Geometry check sheet. Reference: drawing and pictorial views, mm from the part's lowest x, y, z. Round coordinates to 2 decimals unless told otherwise and drop trailing zeros. Order: outer loops, then holes, each group sorted by start corner. A loop starts at its lowest first (then second) coordinate and runs counter-clockwise, first axis right, second up.
(1) Go/stop test with flat-tipped pins: pin 1 (1.8 mm diameter, centred on x = 84, y = 2.5, fed in from -Z); pin 2 (1.8 mm diameter, centred on y = 4, z = 54.5, fed in from -X); pin 3 (1.5 mm diameter, centred on x = 45.5, y = 5, fed in from +Z). Record where each tip stops, or that it passes through.
(2) Sectioned sample at C-C (x = 31). Record the boundary of the cut face in (y, z), plus the area to 3 significant figures.
(3) Material ranges on line 1 along Z through (x, y) = (5, 4); line 2 along X through (y, z) = (2.8, 63.5); line 3 along Z through (x, y) = (51, 1.6), recorded low to high.
(4) Sectioned sample at A-A (y = 2.35). Record the boundary of the cut face in (x, z).
(5) Sectioned sample at B-B (z = 59). Record the boundary of the cut face in (x, y), plus the area to 3 significant figures.
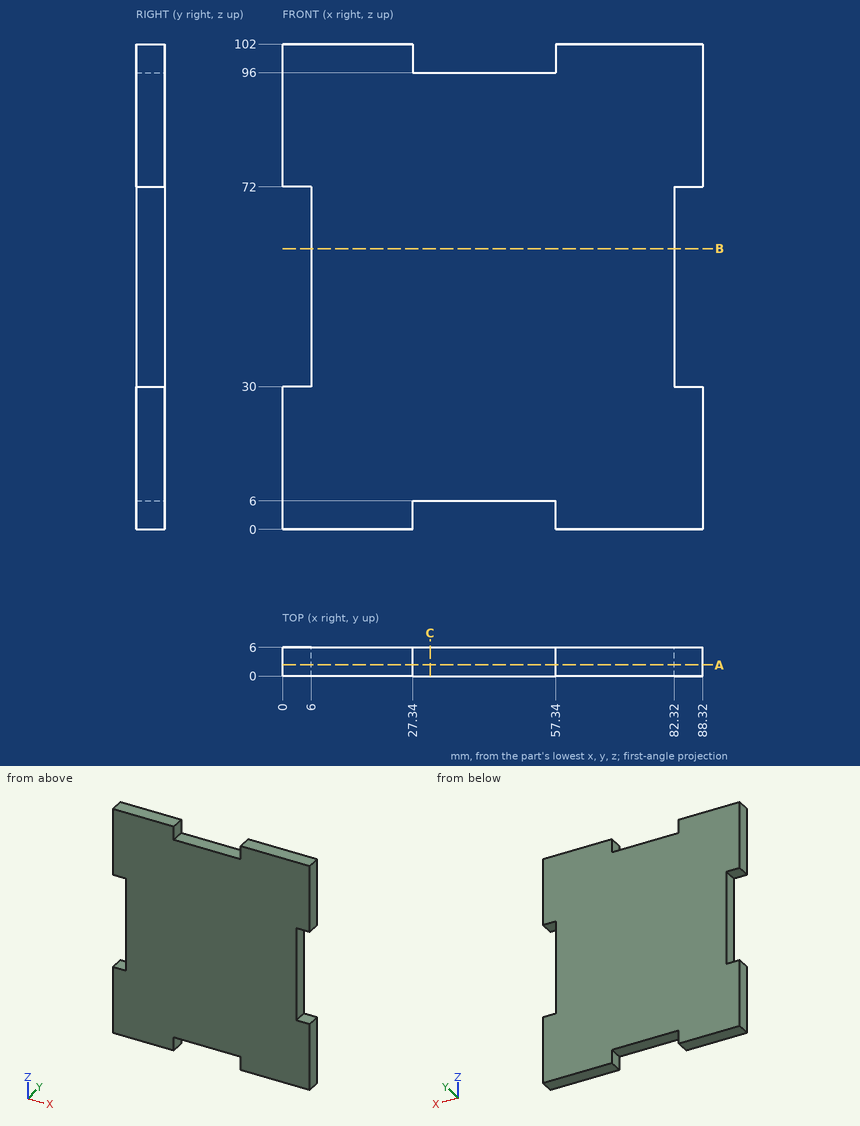
Answer below:
1. pin 1: stops at z = 0
1. pin 2: stops at x = 6
1. pin 3: stops at z = 96
2. outline: (0, 6) - (6, 6) - (6, 96) - (0, 96) - close
2. area: 540 mm2
3. line 1: z = 0 to 30, 72 to 102
3. line 2: x = 6 to 82.32
3. line 3: z = 6 to 96
4. outline: (0, 0) - (27.34, 0) - (27.34, 6) - (57.34, 6) - (57.34, 0) - (88.32, 0) - (88.32, 30) - (82.32, 30) - (82.32, 72) - (88.32, 72) - (88.32, 102) - (57.34, 102) - (57.34, 96) - (27.34, 96) - (27.34, 102) - (0, 102) - (0, 72) - (6, 72) - (6, 30) - (0, 30) - close
5. outline: (6, 0) - (82.32, 0) - (82.32, 6) - (6, 6) - close
5. area: 458 mm2
